```python
from build123d import *

# Parameters (mm, degrees)
SKETCH2_W           = 755.65
SKETCH2_H           = 755.65
BASE_FLANGE1_DEPTH  = 3.175
CUT_EXTRUDE1_DEPTH  = 535.334672162
CUT_EXTRUDE2_DEPTH  = 535.334672162
BREAK_CORNER1_START = -3.175
BREAK_CORNER1_DEPTH = 3.175


# Read off the part's stored shape, not the designer's step: Break-Corner1
# Sheet-metal steps are written as plain solids
with BuildPart() as part:
    # Sketch2 → Base-Flange1 (new body)
    with BuildSketch(Plane(origin=(0, 0, 0), x_dir=(1, 0, 0), z_dir=(0, 1, 0))):
        Rectangle(SKETCH2_W, SKETCH2_H)
    extrude(amount=-BASE_FLANGE1_DEPTH)

    # Sketch3 → Cut-Extrude1 (cut, through all)
    with BuildSketch(Plane(origin=(0, 0, 0), x_dir=(1, 0, 0), z_dir=(0, 1, 0))):
        Polygon((0, -152.664354058), (152.664354058, 0), (0, 152.664354058), (-152.664354058, 0), align=None)
    extrude(amount=-CUT_EXTRUDE1_DEPTH, mode=Mode.SUBTRACT)

    # Sketch4 → Cut-Extrude2 (cut, through all)
    with BuildSketch(Plane(origin=(0, 0, 0), x_dir=(1, 0, 0), z_dir=(0, 1, 0))):
        with BuildLine():
            Line((377.825, 206.375), (352.425, 206.375))
            ThreePointArc((352.425, 206.375), (249.152054608, 249.152054608), (206.375, 352.425))
            Line((206.375, 352.425), (206.375, 377.825))
            Line((206.375, 377.825), (377.825, 377.825))
            Line((377.825, 377.825), (377.825, 206.375))
        make_face()
        with BuildLine():
            Line((206.375, -377.825), (206.375, -352.425))
            ThreePointArc((206.375, -352.425), (249.152054608, -249.152054608), (352.425, -206.375))
            Line((352.425, -206.375), (377.825, -206.375))
            Line((377.825, -206.375), (377.825, -377.825))
            Line((377.825, -377.825), (206.375, -377.825))
        make_face()
        with BuildLine():
            Line((-377.825, -206.375), (-352.425, -206.375))
            ThreePointArc((-352.425, -206.375), (-249.152054608, -249.152054608), (-206.375, -352.425))
            Line((-206.375, -352.425), (-206.375, -377.825))
            Line((-206.375, -377.825), (-377.825, -377.825))
            Line((-377.825, -377.825), (-377.825, -206.375))
        make_face()
        with BuildLine():
            Line((-206.375, 377.825), (-206.375, 352.425))
            ThreePointArc((-206.375, 352.425), (-249.152054608, 249.152054608), (-352.425, 206.375))
            Line((-352.425, 206.375), (-377.825, 206.375))
            Line((-377.825, 206.375), (-377.825, 377.825))
            Line((-377.825, 377.825), (-206.375, 377.825))
        make_face()
    extrude(amount=-CUT_EXTRUDE2_DEPTH, mode=Mode.SUBTRACT)

    # Break-Corner1 outline → Break-Corner1 (cut)
    with BuildSketch(Plane(origin=(0, 0, 0), x_dir=(1, 0, 0), z_dir=(0, 1, 0)).offset(BREAK_CORNER1_START)):
        Polygon((-206.375, 374.65), (-203.2, 377.825), (-206.375, 377.825), align=None)
        Polygon((203.2, 377.825), (206.375, 374.65), (206.375, 377.825), align=None)
        Polygon((377.825, -206.375), (377.825, -203.2), (374.65, -206.375), align=None)
        Polygon((374.65, 206.375), (377.825, 203.2), (377.825, 206.375), align=None)
        Polygon((-374.65, -206.375), (-377.825, -203.2), (-377.825, -206.375), align=None)
        Polygon((-377.825, 203.2), (-374.65, 206.375), (-377.825, 206.375), align=None)
        Polygon((206.375, -374.65), (203.2, -377.825), (206.375, -377.825), align=None)
        Polygon((-203.2, -377.825), (-206.375, -374.65), (-206.375, -377.825), align=None)
    extrude(amount=BREAK_CORNER1_DEPTH, mode=Mode.SUBTRACT)


solid = part.part
```
Can you work these out from the model? Positions are in its coordinate system, mm. A direction names the side the tool comes from. Coordinates: 2 decimals unless noted, no trailing zeros. Loops run counter-clockwise (first coordinate to the right, second up) from the corner with the lowest first, then second, coordinate; pieces in that order, holes last.
1) Imagine slicing it at D-D on x = -263. List the corners of the cut face in (y, z) for me (3 decimals).
2) I need wall thicknesses on probe 1 along X at (y, z) = (-0.2, -48) (3 decimals); probe 2 along X at (y, z) = (-0.8, 15.5) (3 decimals); probe 3 along Z at (x, y) = (-63.5, -3) (3 decimals). Which ranges of each line are inside material? Lowest first, please.
3) Imagine slicing it at C-C on y = -2.6. List the corners of the cut face in (x, z) for me (3 decimals), plus the area to 3 significant figures.
4) Thinking about a two-plate mould opening in X: for faces 3 (the cylindrical face through (-250.294, -1.565, 248.023)), 4 (the cylindrical face through (250.294, -1.565, -248.023)), 5 (the flat face through (75.264, -1.565, 77.401)), which applies, pulls with the +X half, pulls with the -X half, needs draft (parallel to the pull), parting line crosses it, or undercut?
5) For pin 1 (1.6 mm diameter, centred on x = 363, y = -2, fed in from -Z) (3 decimals); pin 2 (1 mm diameter, centred on y = -1, z = 363, fed in from -X) (3 decimals), each with a flat end and sliding along its axis, tell me the tip position at first contact or that it passes through.
6) Which directions (+Z, -Z, +X, -X, +Y, -Y) give clear straight access to the entire face, cutting with the end or side of a thin tool? Please do faces 1 (the flat face through (-75.264, -1.565, -77.401)), 2 (the cylindrical face through (248.023, -1.565, 250.294)).
7) Imagine slicing it at A-A on z = -126.5. List the corners of the cut face in (x, y) for me (3 decimals), plus the area to 3 significant figures.
8) Imagine slicing it at B-B on x = 47. List the corners of the cut face in (y, z) for me (3 decimals), plus the area to 3 significant figures.
Completed:
1. outline: (-3.175, -236.953) - (0, -236.953) - (0, 236.953) - (-3.175, 236.953) - close
2. probe 1: x = -377.825 to -104.664, 104.664 to 377.825
2. probe 2: x = -377.825 to -137.164, 137.164 to 377.825
2. probe 3: z = -377.825 to -89.164, 89.164 to 377.825
3. outline: (-377.825, -203.2) - (-374.65, -206.375) - (-352.425, -206.375) arc R146.05 cw to (-206.375, -352.425) - (-206.375, -374.65) - (-203.2, -377.825) - (203.2, -377.825) - (206.375, -374.65) - (206.375, -352.425) arc R146.05 cw to (352.425, -206.375) - (374.65, -206.375) - (377.825, -203.2) - (377.825, 203.2) - (374.65, 206.375) - (352.425, 206.375) arc R146.05 cw to (206.375, 352.425) - (206.375, 374.65) - (203.2, 377.825) - (-203.2, 377.825) - (-206.375, 374.65) - (-206.375, 352.425) arc R146.05 cw to (-352.425, 206.375) - (-374.65, 206.375) - (-377.825, 203.2) - close; hole (-152.664, 0) - (0, -152.664) - (152.664, 0) - (0, 152.664) - close
3. area: 425,000 mm2
4. face 3: pulls with the -X half
4. face 4: pulls with the +X half
4. face 5: undercut
5. pin 1: stops at z = -206.375
5. pin 2: stops at x = -206.375
6. face 1: +Y, -Y
6. face 2: +Z, +X, +Y, -Y
7. outline: (-377.825, -3.175) - (-26.164, -3.175) - (-26.164, 0) - (-377.825, 0) - close; (26.164, -3.175) - (377.825, -3.175) - (377.825, 0) - (26.164, 0) - close
7. area: 2,230 mm2
8. outline: (-3.175, -377.825) - (0, -377.825) - (0, -105.664) - (-3.175, -105.664) - close; (-3.175, 105.664) - (0, 105.664) - (0, 377.825) - (-3.175, 377.825) - close
8. area: 1,730 mm2
